Model file for the job. Use its own axes, mm. Coordinates: 2 decimals unless noted, no trailing zeros. Order: outer loops, then holes, each group sorted by start corner. A loop starts at its lowest first (then second) coordinate and runs counter-clockwise, first axis right, second up. Notation, with made-up numbers: (64.5, 28.5) -> (97.5, 28.5) arc R30 ccw to (97.5, 65.5) -> close; hole circle Ø4 at (56, -27). An arc over 180 degrees is marked (long way). Use CSV: the item, a comma, the result in double quotes. Start each with the question number.
(1) Cut at C-C on x = -0.25. Write the cut outline in (y, z), plus the area to 3 significant figures.
(2) Pull direction Y, two halves, no side cores. Call faces 1 (the cylindrical face through (0.01, 5.1, -91.57)), 2 (the cylindrical face through (0.01, -18.97, -91.5)), 3 (the cylindrical face through (-0.01, 17.37, 87.27)): pulls with the +Y half, pulls with the -Y half, needs draft (parallel to the pull), parting line crosses it, or undercut.
(3) Pin check, flat tips, straight feed: pin 1 Ø1.9 at (y, z) = (16.4, 78) entering from +X; pin 2 Ø0.5 at (x, z) = (0, -18.5) entering from +Y. Stop position of each tip, or through.
(4) Cut at B-B on y = 16.4. Write the cut outline in (x, z), plus the area to 3 significant figures.
(5) Probe L1, parallel to Z at x = 0.35, y = 16.4; L2, parallel to Y at x = -0.2, z = 78; L3, parallel to Y at x = 0.35, z = -43. List the from-to ranges inside material, lowest first.
(6) Cut at D-D on z = 63.5. Write the cut outline in (x, y).
(7) Cut at A-A on z = 86. Write the cut outline in (x, y), plus the area to 3 significant figures.
Autodesk Inventor part; units mm, degrees
ref_plane "YZ Plane" through (0, 0, 0) normal (1, 0, 0) x (0, 1, 0)
ref_plane "XZ Plane" through (0, 0, 0) normal (0, 1, 0) x (-1, 0, 0)
ref_plane "XY Plane" through (0, 0, 0) normal (0, 0, 1) x (1, 0, 0)
sketch "スケッチ1" plane through (0, 0, 0) normal (1, 0, 0) x (0, 1, 0)
  line L0 (-20.4, 93) -> (20.4, 93)
  line L1 (20.4, 93) -> (20.4, -93)
  line L2 (20.4, -93) -> (-20.4, -93)
  line L3 (-20.4, -93) -> (-20.4, 93)
  line L4 (-20.4, 93) -> (20.4, -93) construction
  line L5 (20.4, 93) -> (-20.4, -93) construction
  line L6 (20.4, 93) -> (-20.4, 93)
  line L7 (-20.4, 93) -> (-20.4, 95)
  line L8 (-20.4, 95) -> (20.4, 95)
  line L9 (20.4, 95) -> (20.4, 93)
  point P0 (0, 0)
  dimension "d0" = 40.8
  dimension "d1" = 186
  dimension "d19" = 2
extrude "プレート1" add sketch "スケッチ1" along normal mid plane 1 contours L0 L1 L2 L3
sketch "スケッチ2" plane through (0.5, 0, 0) normal (1, 0, 0) x (0, 0, -1)
  line L0 (-93, 20.4) -> (93, 20.4)
  line L1 (-93, -20.4) -> (-93, 20.4)
  point P0 (0, 0)
  point P1 (-86, 16.4)
  point P2 (-78, 16.4)
  dimension "d3" = 4
  dimension "d4" = 7
  dimension "d5" = 8
hole "穴1" at (0.5, 16.4, 86) at (0.5, 16.4, 78) direction (-1, 0, 0) diameter 3.2 end through all
sketch "スケッチ3" plane through (-0.5, 0, 0) normal (-1, 0, 0) x (0, 0, 1)
  line L0 (-93, 20.4) -> (-93, -20.4)
  line L1 (-93, 20.4) -> (74, 20.4)
  line L2 (74, 20.4) -> (74, 6.6)
  line L3 (74, 6.6) -> (-93, 6.6)
  line L4 (-93, 6.6) -> (-93, 20.4)
  line L5 (-93, -20.4) -> (93, -20.4)
  line L6 (93, -20.4) -> (93, 20.4)
  point P0 (0, 0)
  point P1 (-93, 6.6)
  dimension "d14" = 19
  dimension "d18" = 13.8
extrude "押し出し1" cut sketch "スケッチ3" against normal blind 10
sketch "スケッチ5" plane through (0.5, 0, 0) normal (1, 0, 0) x (0, 0, -1)
  line L0 (93, -20.4) -> (-93, -20.4)
  line L1 (-93, -20.4) -> (-96.5, -20.4)
  line L2 (-96.5, -20.4) -> (-96.5, 6.6)
  line L3 (-96.5, 6.6) -> (-93, 6.6)
  line L4 (-93, 6.6) -> (-93, -20.4)
  point P0 (0, 0)
  point P1 (-93, 20.4)
  dimension "d34" = 27
  dimension "d35" = 3.5
sheet face with bend "面3" sketch "スケッチ5" thickness 1 toward (-1, 0, 0) bend radius 1
bend "曲げ2"
fillet "コーナーR3" radius 5 3 edges at (0, -20.4, -93) (0, -20.4, 96.5) (0, 6.6, -93)
fillet "コーナーR4" radius 2 2 edges at (0, 6.6, 93) (0, 6.6, 74)
equation "\"d11\" = Thickness"
equation "\"d2\" = Thickness"
equation "\"d28\" = BendRadius"
equation "\"d29\" = BendReliefWidth"
equation "\"d31\" = MinimumRemnant"
equation "\"d30\" = BendReliefDepth"
equation "\"d32\" = TransitionRadius"
equation "\"BendRadius\" = Thickness"
equation "\"BendReliefWidth\" = Thickness"
equation "\"BendReliefDepth\" = 0.5 * Thickness"
equation "\"CornerReliefSize\" = 4 * Thickness"
equation "\"MinimumRemnant\" = 2 * Thickness"
equation "\"TransitionRadius\" = BendRadius"
equation "\"JacobiRadiusSize\" = BendRadius"
equation "\"GapSize\" = Thickness"
properties part number "s_carbon_plate2" material "CFRP"
Outcome:
1,outline,"(-20.4, -88) arc R5 ccw to (-15.4, -93) -> (1.6, -93) arc R5 ccw to (6.6, -88) -> (6.6, 72) arc R2 cw to (8.6, 74) -> (20.4, 74) -> (20.4, 93) -> (8.6, 93) arc R2 cw to (6.6, 95) -> (6.6, 96.5) -> (-15.4, 96.5) arc R5 ccw to (-20.4, 91.5) -> close; hole circle Ø3.2 at (16.4, 78); hole circle Ø3.2 at (16.4, 86)"
1,area,"5,350 mm2"
2,face 1,"pulls with the +Y half"
2,face 2,"pulls with the -Y half"
2,face 3,"undercut"
3,pin 1,"through"
3,pin 2,"y = 6.6"
4,outline,"(-0.5, 74) -> (0.5, 74) -> (0.5, 76.4) -> (-0.5, 76.4) -> close; (-0.5, 79.6) -> (0.5, 79.6) -> (0.5, 84.4) -> (-0.5, 84.4) -> close; (-0.5, 87.6) -> (0.5, 87.6) -> (0.5, 93) -> (-0.5, 93) -> close"
4,area,"12.6 mm2"
5,L1,"74 to 76.4, 79.6 to 84.4, 87.6 to 93"
5,L2,"-20.4 to 14.8, 18 to 20.4"
5,L3,"-20.4 to 6.6"
6,outline,"(-0.5, -20.4) -> (0.5, -20.4) -> (0.5, 6.6) -> (-0.5, 6.6) -> close"
7,outline,"(-0.5, -20.4) -> (0.5, -20.4) -> (0.5, 14.8) -> (-0.5, 14.8) -> close; (-0.5, 18) -> (0.5, 18) -> (0.5, 20.4) -> (-0.5, 20.4) -> close"
7,area,"37.6 mm2"
